Source: CAD feature listing. Evaluate the final solid. Frame: model axes, mm. Give positions to 0.01 mm unless a question says otherwise; leave off trailing zeros. Write each loop counter-clockwise with the first axis right and the second up, starting at its lowest first coordinate (ties: lowest second). Pieces come first, ordered by that corner, then holes. Notation, with made-up numbers: (-18, -30) - (32, -30) arc R24 cw to (32, -20) - close; hole circle Ø4 at (28.5, 72). An arc over 180 degrees is marked (long way). Answer as a JSON object with one key per item and string values. Group by question number.
from build123d import *

# Parameters (mm, degrees)
SKETCH1_W           = 50.5
SKETCH1_H           = 60.2
BOSS_EXTRUDE1_DEPTH = 3.95
FILLET1_RADIUS      = 3.95
FILLET1_LENGTH      = 60.2
FILLET2_RADIUS      = 3.95
FILLET2_LENGTH      = 60.2


with BuildPart() as part:
    # Sketch1 → Boss-Extrude1 (new, symmetric)
    with BuildSketch(Plane.XY):
        Rectangle(SKETCH1_W, SKETCH1_H)
    extrude(amount=BOSS_EXTRUDE1_DEPTH, both=True)

    # Fillet1: full round fillet: the end face becomes a half cylinder, R = half its width
    fillet1_face = Plane((-25.25, 0, 0), x_dir=(0, 1, 0), z_dir=(-1, 0, 0))  # on the end face: x along it, z out of the body
    fillet1_slab = fillet1_face.offset(-FILLET1_RADIUS / 2) * Box(FILLET1_LENGTH, 2 * FILLET1_RADIUS, FILLET1_RADIUS, mode=Mode.PRIVATE)  # the body's end, R deep
    fillet1_round = Plane((-21.3, 0, 0), x_dir=(-1, 0, 0), z_dir=(0, 1, 0)) * Cylinder(FILLET1_RADIUS, FILLET1_LENGTH, mode=Mode.PRIVATE)  # its axis R under the face
    add(fillet1_slab - fillet1_round, mode=Mode.SUBTRACT)

    # Fillet2: full round fillet: the end face becomes a half cylinder, R = half its width
    fillet2_face = Plane((25.25, 0, 0), x_dir=(0, -1, 0), z_dir=(1, 0, 0))  # on the end face: x along it, z out of the body
    fillet2_slab = fillet2_face.offset(-FILLET2_RADIUS / 2) * Box(FILLET2_LENGTH, 2 * FILLET2_RADIUS, FILLET2_RADIUS, mode=Mode.PRIVATE)  # the body's end, R deep
    fillet2_round = Plane((21.3, 0, 0), x_dir=(1, 0, 0), z_dir=(0, -1, 0)) * Cylinder(FILLET2_RADIUS, FILLET2_LENGTH, mode=Mode.PRIVATE)  # its axis R under the face
    add(fillet2_slab - fillet2_round, mode=Mode.SUBTRACT)


solid = part.part
Q1. Section A-A on y = -9. Return the cut outline in (x, z).
Q2. Ray query, probe 1 along X at (y, z) = (-14.5, -0.25); probe 2 along X at (y, z) = (-3.5, -1.25); probe 3 along Z at (x, y) = (22, 14). Return the intervals inside material, ascending. Write a range as [from, to].
Q3. First-contact query: pin 1 Ø2 at (y, z) = (19.5, 2.5) entering from -X; pin 2 Ø3 at (y, z) = (6, -2.5) entering from -X. Flat tips, straight axial feed; report the tip coordinate or a pass-through.
Taken from the geometry:
{
 "1": {"outline": "(-21.3, -3.95) - (21.3, -3.95) arc R3.95 ccw to (21.3, 3.95) - (-21.3, 3.95) arc R3.95 ccw to start"},
 "2": {"probe 1": "x = [-25.24, 25.24]", "probe 2": "x = [-25.05, 25.05]", "probe 3": "z = [-3.89, 3.89]"},
 "3": {"pin 1": "stops at x = -24.95", "pin 2": "stops at x = -25.12"}
}
